Model file for the job. Use its own axes, mm. Round coordinates to 2 decimals unless told otherwise and drop trailing zeros. Loops run counter-clockwise (first coordinate to the right, second up) from the corner with the lowest first, then second, coordinate; pieces in that order, holes last. Notation, with made-up numbers: M 85.25,64 L 103.25,64 A27 cw 103.25,82 Z; hole C 48.25,25.25 d7. An arc over 180 degrees is marked long. Use a Markdown table: item, result. Add a question column.
Q1. Cut at C-C (z = 305). Give the cut face in (x, y), plus the area to 3 significant figures.
Q2. Probe line 1 (Z direction, x = -175, y = 1); line 2 (X direction, y = 0.55, z = 317.5); line 3 (Z direction, x = -82.5, y = 1.4). List the from-to ranges inside material, lowest first. Write a range as from..to.
Q3. Pin check, flat tips, straight feed: pin 1 (4.5 mm diameter, centred on x = -19.02, z = 235.14, fed in from -Y); pin 2 (0.5 mm diameter, centred on y = 0.5, z = 320.5, fed in from +X); pin 3 (0.5 mm diameter, centred on x = -105, y = 0.5, fed in from +Z). Stop position of each tip, or through.
Q4. Cut at B-B (y = 0.25). State how many separate pieces and enclosed holes the cut face has, plus the area to 3 significant figures.
Q5. Cut at A-A (x = -88.5). Give the cut face in (y, z).
from build123d import *

# Parameters (mm, degrees)
SKETCH1_R        = 1.8
SKETCH1_R_2      = 1.85915493
EXTRUSION1_DEPTH = 1.6
FILLET1_R        = 1
FILLET2_R        = 4
FILLET3_R        = 3
FILLET4_R        = 3
FILLET5_R        = 2
FILLET6_R        = 2
FILLET7_R        = 3
FILLET8_R        = 3
FILLET9_R        = 2
FILLET10_R       = 2
FILLET11_R       = 3


with BuildPart() as part:
    # Sketch1 → Extrusion1 (new body)
    with BuildSketch(Plane(origin=(0, 0, 0), x_dir=(-1, 0, 0), z_dir=(0, 1, 0))):
        Polygon((74.087520418, 321.088295015), (70.369210559, 327.285477572), (45.580478165, 327.285477572), (45.580478165, 312.412238135), (23.246043749, 290.934342561), (26.682507041, 287.360833055), (12.735407819, 253.538985229), (9.017097883, 253.538985229), (9.017097883, 226.891111382), (9.017097883, 200.243237534), (12.735407819, 200.243237534), (26.682507041, 166.421389708), (23.246043749, 162.847880202), (45.580478165, 141.369984628), (45.580478165, 126.496745191), (70.369210559, 126.496745191), (74.087520418, 132.693927748), (97.636816193, 132.693927748), (121.186111968, 132.693927748), (124.904421827, 126.496745191), (149.693154221, 126.496745191), (149.693154221, 141.369984628), (172.027588636, 162.847880202), (168.591125345, 166.421389708), (182.538224567, 200.243237534), (186.256534503, 200.243237534), (186.256534503, 226.891111382), (186.256534503, 253.538985229), (182.538224567, 253.538985229), (168.591125345, 287.360833055), (172.027588636, 290.934342561), (149.693154221, 312.412238135), (149.693154221, 327.285477572), (124.904421827, 327.285477572), (121.186111968, 321.088295015), (97.636816193, 321.088295015), align=None)
        with Locations((176.256534503, 218.641111382)):
            Circle(SKETCH1_R, mode=Mode.SUBTRACT)
        with Locations((176.256534503, 235.141111382)):
            Circle(SKETCH1_R, mode=Mode.SUBTRACT)
        with Locations((19.017097883, 218.641111382)):
            Circle(SKETCH1_R, mode=Mode.SUBTRACT)
        with Locations((19.017097883, 235.141111382)):
            Circle(SKETCH1_R, mode=Mode.SUBTRACT)
        with Locations((51.777661187, 316.130534525)):
            Circle(SKETCH1_R_2, mode=Mode.SUBTRACT)
        with Locations((143.495971199, 137.651688238)):
            Circle(SKETCH1_R_2, mode=Mode.SUBTRACT)
        with Locations((143.495971199, 316.130534525)):
            Circle(SKETCH1_R_2, mode=Mode.SUBTRACT)
        with Locations((51.777661187, 137.651688238)):
            Circle(SKETCH1_R_2, mode=Mode.SUBTRACT)
    extrude(amount=EXTRUSION1_DEPTH)

    # Fillet1
    fillet1_edges = [part.edges().sort_by_distance(p)[0] for p in [
        (-121.186111968, 0.8, 321.088295015),
        (-121.186111968, 0.8, 132.693927748),
        (-74.087520418, 0.8, 132.693927748),
        (-74.087520418, 0.8, 321.088295015),
    ]]
    fillet(fillet1_edges, radius=FILLET1_R)

    # Fillet2
    fillet2_edges = [part.edges().sort_by_distance(p)[0] for p in [
        (-149.693154221, 0.8, 327.285477572),
        (-149.693154221, 0.8, 126.496745191),
        (-45.580478165, 0.8, 126.496745191),
        (-45.580478165, 0.8, 327.285477572),
    ]]
    fillet(fillet2_edges, radius=FILLET2_R)

    # Fillet3
    fillet3_edges = [part.edges().sort_by_distance(p)[0] for p in [
        (-149.693154221, 0.8, 312.412238135),
        (-149.693154221, 0.8, 141.369984628),
        (-45.580478165, 0.8, 141.369984628),
        (-45.580478165, 0.8, 312.412238135),
    ]]
    fillet(fillet3_edges, radius=FILLET3_R)

    # Fillet4
    fillet4_edges = [part.edges().sort_by_distance(p)[0] for p in [
        (-172.027588636, 0.8, 290.934342561),
    ]]
    fillet(fillet4_edges, radius=FILLET4_R)

    # Fillet5
    fillet5_edges = [part.edges().sort_by_distance(p)[0] for p in [
        (-168.591125345, 0.8, 287.360833055),
    ]]
    fillet(fillet5_edges, radius=FILLET5_R)

    # Fillet6
    fillet6_edges = [part.edges().sort_by_distance(p)[0] for p in [
        (-26.682507041, 0.8, 287.360833055),
    ]]
    fillet(fillet6_edges, radius=FILLET6_R)

    # Fillet7
    fillet7_edges = [part.edges().sort_by_distance(p)[0] for p in [
        (-23.246043749, 0.8, 290.934342561),
    ]]
    fillet(fillet7_edges, radius=FILLET7_R)

    # Fillet8
    fillet8_edges = [part.edges().sort_by_distance(p)[0] for p in [
        (-172.027588636, 0.8, 162.847880202),
        (-23.246043749, 0.8, 162.847880202),
    ]]
    fillet(fillet8_edges, radius=FILLET8_R)

    # Fillet9
    fillet9_edges = [part.edges().sort_by_distance(p)[0] for p in [
        (-168.591125345, 0.8, 166.421389708),
        (-26.682507041, 0.8, 166.421389708),
    ]]
    fillet(fillet9_edges, radius=FILLET9_R)

    # Fillet10
    fillet10_edges = [part.edges().sort_by_distance(p)[0] for p in [
        (-182.538224567, 0.8, 253.538985229),
        (-182.538224567, 0.8, 200.243237534),
        (-12.735407819, 0.8, 200.243237534),
        (-12.735407819, 0.8, 253.538985229),
    ]]
    fillet(fillet10_edges, radius=FILLET10_R)

    # Fillet11
    fillet11_edges = [part.edges().sort_by_distance(p)[0] for p in [
        (-186.256534503, 0.8, 200.243237534),
        (-186.256534503, 0.8, 253.538985229),
        (-9.017097883, 0.8, 253.538985229),
        (-9.017097883, 0.8, 200.243237534),
    ]]
    fillet(fillet11_edges, radius=FILLET11_R)


solid = part.part
Checked values:
| question | item | result |
|---|---|---|
| 1 | outline | M -157.4,0 L -37.87,0 L -37.87,1.6 L -157.4,1.6 Z |
| 1 | area | 191 mm^2 |
| 2 | line 1 | z = 181.96..217.35, 219.93..233.85, 236.43..271.82 |
| 2 | line 2 | x = -149.69..-144.75, -142.24..-53.04, -50.52..-45.58 |
| 2 | line 3 | z = 132.69..321.09 |
| 3 | pin 1 | stops at y = 0 |
| 3 | pin 2 | stops at x = -45.58 |
| 3 | pin 3 | stops at z = 321.09 |
| 4 | separate pieces | 1 |
| 4 | enclosed holes | 8 |
| 4 | area | 28,800 mm^2 |
| 5 | outline | M 0,132.69 L 1.6,132.69 L 1.6,321.09 L 0,321.09 Z |
